The listing builds one solid part. Answer for the finished solid, in the listing's coordinates (mm). A direction names the side the tool comes from. Coordinates: 2 decimals unless noted, no trailing zeros. Loops run counter-clockwise (first coordinate to the right, second up) from the corner with the lowest first, then second, coordinate; pieces in that order, holes last. Notation, with made-up numbers: (11, 22) - (43, 22) arc R25 cw to (43, 38) - close; hole circle Ø4 at (35, -23). An arc over 180 degrees is marked (long way). Put each result on its own line as item: value.
```python
from build123d import *

# Parameters (mm, degrees)
SKETCH1_W              = 165.1
SKETCH1_H              = 47.498
BOSS_EXTRUDE1_DEPTH    = 22.098
F_10_32_TAPPED_HOLE1_D = 4.0386


with BuildPart() as part:
    # Sketch1 → Boss-Extrude1 (new body)
    with BuildSketch(Plane(origin=(0, 0, 0), x_dir=(0, 0, -1), z_dir=(1, 0, 0))):
        Rectangle(SKETCH1_W, SKETCH1_H)
        with BuildLine():
            Line((-67.5752522, 6.6675), (67.5752522, 6.6675))
            ThreePointArc((67.5752522, 6.6675), (74.2427522, 0), (67.5752522, -6.6675))
            Line((67.5752522, -6.6675), (-67.5752522, -6.6675))
            ThreePointArc((-67.5752522, -6.6675), (-74.2427522, 0), (-67.5752522, 6.6675))
        make_face(mode=Mode.SUBTRACT)
    extrude(amount=BOSS_EXTRUDE1_DEPTH)

    # #10-32 Tapped Hole1 (through all)
    with Locations(Plane(origin=(22.098, 0, 0), x_dir=(0, 0, -1), z_dir=(1, 0, 0))):
        with Locations((-76.2, 17.399), (-76.2, -17.399), (0, -17.399), (76.2, -17.399), (76.2, 17.399), (0, 17.399)):
            Hole(F_10_32_TAPPED_HOLE1_D / 2)


solid = part.part
```
1) The part is cut by section A-A (y = 0). Give the vertices of the cut face in (x, z).
Found:
outline: (0, -82.55) - (22.1, -82.55) - (22.1, -74.24) - (0, -74.24) - close; (0, 74.24) - (22.1, 74.24) - (22.1, 82.55) - (0, 82.55) - close
2) The part is cut by section B-B (z = -76.2). Give the vertices of the cut face in (x, y).
Found:
outline: (0, -23.75) - (22.1, -23.75) - (22.1, -19.42) - (0, -19.42) - close; (0, -15.38) - (22.1, -15.38) - (22.1, 15.38) - (0, 15.38) - close; (0, 19.42) - (22.1, 19.42) - (22.1, 23.75) - (0, 23.75) - close
3) The part is cut by section D-D (z = 34.5). Give the vertices of the cut face in (x, y).
Found:
outline: (0, -23.75) - (22.1, -23.75) - (22.1, -6.67) - (0, -6.67) - close; (0, 6.67) - (22.1, 6.67) - (22.1, 23.75) - (0, 23.75) - close
4) This flat-tipped pin is pushed along its axis until it touches: pin 1 (5.5 mm diameter, centred on y = -17.399, z = 76.2, fed in from +X). Where does it stop, or does it pass through?
Found:
pin 1: stops at x = 22.1
5) For faces 1 (the face through (11, -23.749, 1)), 2 (the face through (10.89, 0.15, -74.24)), determine the directions among +Z, -Z, +X, -X, +Y, -Y from which every point of the face is accessible in a straight line to the end or side of a thin tool.
Found:
face 1: +Z, -Z, +X, -X, -Y
face 2: +X, -X
6) For a pull along Z with two mould halves and no side action, classify faces 3 (the face through (10.894, -17.31, 74.183)), 4 (the face through (11, 23.749, 1)), 5 (the face through (11, 0, -82.55)) as pulls with the +Z half, pulls with the -Z half, needs draft (parallel to the pull), parting line crosses it, or undercut.
Found:
face 3: undercut
face 4: needs draft
face 5: pulls with the -Z half
7) Straight lines are drawn through the part: L1, parallel to Y at x = 15.25, z = 76.2; L2, parallel to Y at x = 17.25, z = 0; L3, parallel to Y at x = 13.75, z = 51.5. For each, find the intervals that lie inside material, in ascending order. Write a range as [from, to].
Found:
L1: y = [-23.75, -19.42], [-15.38, 15.38], [19.42, 23.75]
L2: y = [-23.75, -19.42], [-15.38, -6.67], [6.67, 15.38], [19.42, 23.75]
L3: y = [-23.75, -6.67], [6.67, 23.75]
8) The part is cut by section C-C (z = 0). Give the vertices of the cut face in (x, y), and give its area (3 significant figures).
Found:
outline: (0, -23.75) - (22.1, -23.75) - (22.1, -19.42) - (0, -19.42) - close; (0, -15.38) - (22.1, -15.38) - (22.1, -6.67) - (0, -6.67) - close; (0, 6.67) - (22.1, 6.67) - (22.1, 15.38) - (0, 15.38) - close; (0, 19.42) - (22.1, 19.42) - (22.1, 23.75) - (0, 23.75) - close
area: 576 mm^2
